Verification items for the finished model (mm, model axes). Face numbers are marked on the shaded views. Give positions to 0.01 mm unless a question says otherwise; leave off trailing zeros. Order: outer loops, then holes, each group sorted by start corner. A loop starts at its lowest first (then second) coordinate and runs counter-clockwise, first axis right, second up. Notation, with made-up numbers: (31.25, 23) - (65.25, 23) arc R9 ccw to (65.25, 34) - close; hole circle Ø6 at (-16, 81.5). An arc over 180 degrees is marked (long way). Answer as a JSON object with one key per item and string values. Group by question number.
(1) Mould release check, pull along X, two halves, no side actions. Record for the marked faces 1, 2 and 3: +X half, -X half, draft (parallel to the pull), parting line (faces both ways), or undercut.
(2) Section check C-C (z = 41.5). Record the boundary of the cut face in (x, y), then the cut area to 3 significant figures.
(3) Section check A-A (x = 0). Record the boundary of the cut face in (y, z), then the cut area to 3 significant figures.
(4) Depth check by flat-ended pin: pin 1 Ø8 at (x, z) = (10.5, 44) entering from -Y; pin 2 Ø8 at (x, z) = (-10, 45.5) entering from +Y; pin 3 Ø10 at (x, z) = (-8, 35) entering from +Y. Enter the tip coordinate at first touch or a pass-through.
(5) Thickness scan on line 1 (X direction, y = 0, z = 39.75); line 2 (Y direction, x = -10, z = 42.5). Record the ranges inside material, lowest first.
```python
from build123d import *

# Parameters (mm, degrees)
ESQUISSE1_R             = 24.25
ESQUISSE1_R_2           = 20.25
BOSS_EXTRU_1_DEPTH      = 48
CHANFREIN1_SIZE         = 3
ESQUISSE2_R             = 24.25
ENL_V_MAT_EXTRU_1_DEPTH = 30


with BuildPart() as part:
    # Esquisse1 → Boss.-Extru.1 (new body)
    with BuildSketch(Plane.XY):
        Circle(ESQUISSE1_R)
        Circle(ESQUISSE1_R_2, mode=Mode.SUBTRACT)
    extrude(amount=BOSS_EXTRU_1_DEPTH)

    # Chanfrein1
    chanfrein1_edges = [part.edges().sort_by_distance(p)[0] for p in [
        (-20.25, 0, 48),
    ]]
    chamfer(chanfrein1_edges, length=CHANFREIN1_SIZE)

    # Esquisse2 → Enlèv. mat.-Extru.1 (cut)
    with BuildSketch(Plane(origin=(0, 0, 0), x_dir=(-1, 0, 0), z_dir=(0, 0, -1))):
        Circle(ESQUISSE2_R)
    extrude(amount=-ENL_V_MAT_EXTRU_1_DEPTH, mode=Mode.SUBTRACT)


solid = part.part
```
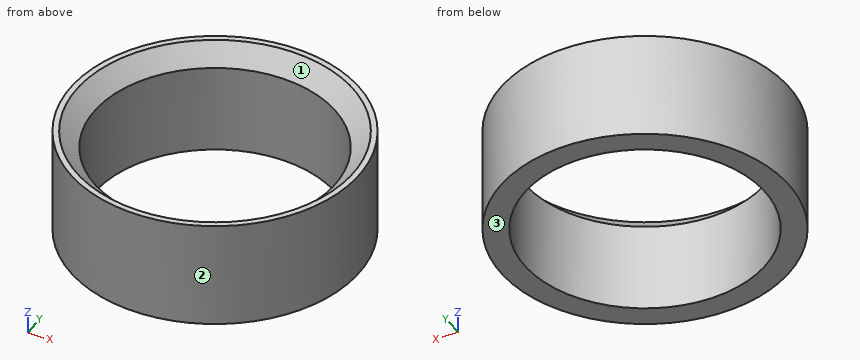
Solutions:
{
 "1": {"face 1": "undercut", "face 2": "parting line", "face 3": "draft"},
 "2": {"outline": "circle Ø48.5 at (0, 0); hole circle Ø40.5 at (0, 0)", "area": "559 mm2"},
 "3": {"outline": "(-24.25, 30) - (-20.25, 30) - (-20.25, 45) - (-23.25, 48) - (-24.25, 48) - close; (20.25, 30) - (24.25, 30) - (24.25, 48) - (23.25, 48) - (20.25, 45) - close", "area": "135 mm2"},
 "4": {"pin 1": "stops at y = -23.36", "pin 2": "stops at y = 23.5", "pin 3": "stops at y = 24.06"},
 "5": {"line 1": "x = -24.25 to -20.25, 20.25 to 24.25", "line 2": "y = -22.09 to -17.61, 17.61 to 22.09"}
}
